Read the model definition and answer for the solid it produces. Units are mm, in the model's axes. A direction names the side the tool comes from. Round coordinates to 2 decimals unless told otherwise and drop trailing zeros. Order: outer loops, then holes, each group sorted by start corner. A loop starts at its lowest first (then second) coordinate and runs counter-clockwise, first axis right, second up. Notation, with made-up numbers: (66.5, 69.25) - (120.5, 69.25) arc R17 ccw to (120.5, 101.25) - close; hole circle Ø2 at (79, -30.5). An arc over 180 degrees is marked (long way). Answer as a JSON object with one key per item and string values. Group by question number.
Q1. Consider line 1 (X direction, y = -1.2, z = 512); line 2 (X direction, y = 2.65, z = 941); line 3 (X direction, y = -2.75, z = 881.5). Determine where each line is inside the solid, lowest interval first.
Q2. A tool of negligible diameter and unlimited length cuts with its end or side. For faces 4 (the flat face through (13, 1, 510)), 5 (the flat face through (-40, 0, 750)), from which of +Z, -Z, +X, -X, +Y, -Y can it reach the whole face along a straight path? Write none if from no direction.
Q3. Given pin 1 Ø5 at (x, z) = (-15, 913.6) entering from -Y; pin 2 Ø3 at (x, z) = (35, 588.5) entering from -Y, each flat-ended and moving along its own axis, determine where each tip first touches the part or whether it passes through.
Q4. A cutting plane is placed at A-A on z = 563.5. Determine the outline of the cut face in (x, y).
Q5. The mould has two halves that part along X. Classify faces 1 (the flat face through (-1, 0, 1000)), 2 (the flat face through (13, 1, 882)), 3 (the flat face through (40, 0, 750)): pulls with the +X half, pulls with the -X half, needs draft (parallel to the pull), parting line crosses it, or undercut.
```python
from build123d import *

# Parameters (mm, degrees)
SKETCH_1_W                  = 80
SKETCH_1_H                  = 8
EXTRUDE_1_DEPTH             = 1000
SKETCH_3_R                  = 4
CUT_EXTRUDE_1_DEPTH         = 5
SKETCH_4_R                  = 2.25
CUT_EXTRUDE_2_DEPTH         = 5
SKETCH_5_R                  = 2.25
CUT_EXTRUDE_3_DEPTH         = 8
PATTERN_LINEAR_1_COUNT      = 2
PATTERN_LINEAR_1_PITCH      = 30
PATTERN_LINEAR_1_COUNT_DIR2 = 2
PATTERN_LINEAR_1_PITCH_DIR2 = 30
SKETCH_6_R                  = 4
CUT_EXTRUDE_4_DEPTH         = 5
PATTERN_LINEAR_2_COUNT      = 2
PATTERN_LINEAR_2_PITCH      = 30
PATTERN_LINEAR_2_COUNT_DIR2 = 2
PATTERN_LINEAR_2_PITCH_DIR2 = 30
PATTERN_LINEAR_11_COUNT     = 2
PATTERN_LINEAR_11_PITCH     = 10
CUT_EXTRUDE_8_DEPTH         = 4
CUT_EXTRUDE_9_DEPTH         = 5
PATTERN_LINEAR_5_COUNT      = 2
PATTERN_LINEAR_5_PITCH      = 610
PATTERN_LINEAR_6_COUNT      = 2
PATTERN_LINEAR_6_PITCH      = 225
PATTERN_LINEAR_7_COUNT      = 2
PATTERN_LINEAR_7_PITCH      = 385
SKETCH_13_R                 = 1.5
CUT_EXTRUDE_10_DEPTH        = 8
SKETCH_14_R                 = 3
CUT_EXTRUDE_11_DEPTH        = 4
PATTERN_LINEAR_8_COUNT      = 2
PATTERN_LINEAR_8_PITCH      = 927
SKETCH_15_R                 = 1.65
CUT_EXTRUDE_12_DEPTH        = 10
PATTERN_LINEAR_9_COUNT      = 5
PATTERN_LINEAR_9_PITCH      = 60
SKETCH_16_R                 = 1.65
CUT_EXTRUDE_13_DEPTH        = 10
PATTERN_LINEAR_10_COUNT     = 5
PATTERN_LINEAR_10_PITCH     = 60
SKETCH_17_W                 = 80
SKETCH_17_H                 = 507
CUT_EXTRUDE_14_DEPTH        = 10


with BuildPart() as part:
    # Эскиз1 → Бобышка-Вытянуть1 (new body)
    with BuildSketch(Plane.XY):
        Rectangle(SKETCH_1_W, SKETCH_1_H)
    extrude(amount=EXTRUDE_1_DEPTH)

    # Эскиз3 → Вырез-Вытянуть1 (cut)
    with BuildSketch(Plane.XZ.offset(4)):
        with Locations(Location((15, 512, 0), (0, 0, 270))):
            Circle(SKETCH_3_R)
        with Locations(Location((-15, 512, 0), (0, 0, 270))):
            Circle(SKETCH_3_R)
    cut_extrude_1 = extrude(amount=-CUT_EXTRUDE_1_DEPTH, mode=Mode.SUBTRACT)

    # Эскиз4 → Вырез-Вытянуть2 (cut)
    with BuildSketch(Plane.XZ.offset(-1)):
        with Locations(Location((-15, 512, 0), (0, 0, 270))):
            Circle(SKETCH_4_R)
        with Locations(Location((15, 512, 0), (0, 0, 270))):
            Circle(SKETCH_4_R)
    cut_extrude_2 = extrude(amount=-CUT_EXTRUDE_2_DEPTH, mode=Mode.SUBTRACT)

    # Эскиз5 → Вырез-Вытянуть3 (cut)
    with BuildSketch(Plane.XZ.offset(4)):
        with Locations(Location((-15, 913.6, 0), (0, 0, 270))):
            Circle(SKETCH_5_R)
    cut_extrude_3 = extrude(amount=-CUT_EXTRUDE_3_DEPTH, mode=Mode.SUBTRACT)

    # Линейный массив1: Cut-Extrude 3 2 × 2
    with Locations(*[(i * PATTERN_LINEAR_1_PITCH, 0, -j * PATTERN_LINEAR_1_PITCH_DIR2) for i in range(PATTERN_LINEAR_1_COUNT) for j in range(PATTERN_LINEAR_1_COUNT_DIR2) if (i, j) != (0, 0)]):
        add(cut_extrude_3, mode=Mode.SUBTRACT)

    # Эскиз6 → Вырез-Вытянуть4 (cut)
    with BuildSketch(Plane.XZ.offset(4)):
        with Locations(Location((-15, 913.6, 0), (0, 0, 270))):
            Circle(SKETCH_6_R)
    cut_extrude_4 = extrude(amount=-CUT_EXTRUDE_4_DEPTH, mode=Mode.SUBTRACT)

    # Линейный массив2: Cut-Extrude 4 2 × 2
    with Locations(*[(i * PATTERN_LINEAR_2_PITCH, 0, -j * PATTERN_LINEAR_2_PITCH_DIR2) for i in range(PATTERN_LINEAR_2_COUNT) for j in range(PATTERN_LINEAR_2_COUNT_DIR2) if (i, j) != (0, 0)]):
        add(cut_extrude_4, mode=Mode.SUBTRACT)

    # Линейный массив11: Вырез-Вытянуть1, Вырез-Вытянуть2 ×2
    with Locations(*[(0, 0, i * PATTERN_LINEAR_11_PITCH) for i in range(1, PATTERN_LINEAR_11_COUNT)]):
        add(cut_extrude_1, mode=Mode.SUBTRACT)
        add(cut_extrude_2, mode=Mode.SUBTRACT)

    # Эскиз11 → Вырез-Вытянуть8 (cut)
    with BuildSketch(Plane.XZ.offset(4)):
        with BuildLine():
            Line((37.5, 220), (37.5, 170))
            ThreePointArc((37.5, 170), (34.5, 167), (31.5, 170))
            Line((31.5, 170), (31.5, 220))
            ThreePointArc((31.5, 220), (34.5, 223), (37.5, 220))
        make_face()
    cut_extrude_8 = extrude(amount=-CUT_EXTRUDE_8_DEPTH, mode=Mode.SUBTRACT)

    # Эскиз12 → Вырез-Вытянуть9 (cut)
    with BuildSketch(Plane(origin=(0, 0, 0), x_dir=(-1, 0, 0), z_dir=(0, -1, 0))):
        with BuildLine():
            Line((-36.25, -218.75), (-36.25, -171.25))
            ThreePointArc((-36.25, -171.25), (-34.5, -169.5), (-32.75, -171.25))
            Line((-32.75, -171.25), (-32.75, -218.75))
            ThreePointArc((-32.75, -218.75), (-34.5, -220.5), (-36.25, -218.75))
        make_face()
    cut_extrude_9 = extrude(amount=-CUT_EXTRUDE_9_DEPTH, mode=Mode.SUBTRACT)

    # Линейный массив5: Вырез-Вытянуть8, Вырез-Вытянуть9 ×2
    with Locations(*[(0, 0, i * PATTERN_LINEAR_5_PITCH) for i in range(1, PATTERN_LINEAR_5_COUNT)]):
        add(cut_extrude_8, mode=Mode.SUBTRACT)
        add(cut_extrude_9, mode=Mode.SUBTRACT)

    # Линейный массив6: Вырез-Вытянуть8, Вырез-Вытянуть9 ×2
    with Locations(*[(0, 0, i * PATTERN_LINEAR_6_PITCH) for i in range(1, PATTERN_LINEAR_6_COUNT)]):
        add(cut_extrude_8, mode=Mode.SUBTRACT)
        add(cut_extrude_9, mode=Mode.SUBTRACT)

    # Линейный массив7: Вырез-Вытянуть8, Вырез-Вытянуть9 ×2
    with Locations(*[(0, 0, i * PATTERN_LINEAR_7_PITCH) for i in range(1, PATTERN_LINEAR_7_COUNT)]):
        add(cut_extrude_8, mode=Mode.SUBTRACT)
        add(cut_extrude_9, mode=Mode.SUBTRACT)

    # Эскиз13 → Вырез-Вытянуть10 (cut)
    with BuildSketch(Plane.XZ.offset(4)):
        with Locations(Location((-14, 59, 0), (0, 0, 270))):
            Circle(SKETCH_13_R)
        with Locations(Location((-14, 14, 0), (0, 0, 270))):
            Circle(SKETCH_13_R)
    cut_extrude_10 = extrude(amount=-CUT_EXTRUDE_10_DEPTH, mode=Mode.SUBTRACT)

    # Эскиз14 → Вырез-Вытянуть11 (cut)
    with BuildSketch(Plane.XZ.offset(4)):
        with Locations(Location((-14, 59, 0), (0, 0, 270))):
            Circle(SKETCH_14_R)
        with Locations(Location((-14, 14, 0), (0, 0, 270))):
            Circle(SKETCH_14_R)
    cut_extrude_11 = extrude(amount=-CUT_EXTRUDE_11_DEPTH, mode=Mode.SUBTRACT)

    # Линейный массив8: Вырез-Вытянуть10, Вырез-Вытянуть11 ×2
    with Locations(*[(0, 0, i * PATTERN_LINEAR_8_PITCH) for i in range(1, PATTERN_LINEAR_8_COUNT)]):
        add(cut_extrude_10, mode=Mode.SUBTRACT)
        add(cut_extrude_11, mode=Mode.SUBTRACT)

    # Эскиз15 → Вырез-Вытянуть12 (cut)
    with BuildSketch(Plane.XZ.offset(4)):
        with Locations(Location((0, 421.45, 0), (0, 0, 270))):
            Circle(SKETCH_15_R)
    cut_extrude_12 = extrude(amount=-CUT_EXTRUDE_12_DEPTH, mode=Mode.SUBTRACT)

    # Линейный массив9: Вырез-Вытянуть12 ×5
    with Locations(*[(0, 0, -i * PATTERN_LINEAR_9_PITCH) for i in range(1, PATTERN_LINEAR_9_COUNT)]):
        add(cut_extrude_12, mode=Mode.SUBTRACT)

    # Эскиз16 → Вырез-Вытянуть13 (cut)
    with BuildSketch(Plane.XZ.offset(4)):
        with Locations(Location((0, 578.55, 0), (0, 0, 270))):
            Circle(SKETCH_16_R)
    cut_extrude_13 = extrude(amount=-CUT_EXTRUDE_13_DEPTH, mode=Mode.SUBTRACT)

    # Линейный массив10: Вырез-Вытянуть13 ×5
    with Locations(*[(0, 0, i * PATTERN_LINEAR_10_PITCH) for i in range(1, PATTERN_LINEAR_10_COUNT)]):
        add(cut_extrude_13, mode=Mode.SUBTRACT)

    # Эскиз17 → Вырез-Вытянуть14 (cut)
    with BuildSketch(Plane.XZ.offset(4)):
        with Locations((0, 253.5)):
            Rectangle(SKETCH_17_W, SKETCH_17_H)
    extrude(amount=-CUT_EXTRUDE_14_DEPTH, mode=Mode.SUBTRACT)


solid = part.part
```
Result set:
{
 "1": {"line 1": "x = -40 to -19, -11 to 11, 19 to 40", "line 2": "x = -40 to -15.5, -12.5 to 40", "line 3": "x = -40 to -18.4, -11.6 to 11.6, 18.4 to 40"},
 "2": {"face 4": "-Y", "face 5": "+Z, -Z, -X, +Y, -Y"},
 "3": {"pin 1": "stops at y = 1", "pin 2": "stops at y = 0"},
 "4": {"outline": "(-40, -4) - (31.5, -4) - (31.5, 0) - (32.75, 0) - (32.75, 4) - (-40, 4) - close; (36.25, 0) - (37.5, 0) - (37.5, -4) - (40, -4) - (40, 4) - (36.25, 4) - close"},
 "5": {"face 1": "needs draft", "face 2": "undercut", "face 3": "pulls with the +X half"}
}
